Autodesk Inventor part; units mm, degrees
ref_plane "YZ Plane" through (0, 0, 0) normal (1, 0, 0) x (0, 1, 0)
ref_plane "XZ Plane" through (0, 0, 0) normal (0, 1, 0) x (-1, 0, 0)
ref_plane "XY Plane" through (0, 0, 0) normal (0, 0, 1) x (1, 0, 0)
sketch "Sketch1" plane through (0, 0, 0) normal (0, 1, 0) x (-1, 0, 0)
  line L0 (40.7614, 52.7865) -> (-35.4386, 52.7865)
  line L1 (-35.4386, 52.7865) -> (-35.4386, -99.6135)
  line L2 (-35.4386, -99.6135) -> (40.7614, -99.6135)
  line L3 (40.7614, -99.6135) -> (40.7614, 52.7865)
  circle A0 centre (2.6614, -23.4135) radius 25.4
  point P0 (0, 0)
  dimension "d0" = 152.4
  dimension "d1" = 76.2
  dimension "d2" = 50.8
  dimension "d5" = 76.2
  dimension "d6" = 38.1
extrude "Extrusion1" add sketch "Sketch1" along normal blind 12.7
sketch "Sketch2" plane through (-40.7614, 0, 52.7865) normal (0, 0, 1) x (1, 0, 0)
  line L0 (18.073, 9.7491) -> (58.127, 9.7491)
  line L1 (58.127, 9.7491) -> (58.127, 2.9509)
  line L2 (58.127, 2.9509) -> (18.073, 2.9509)
  line L3 (18.073, 2.9509) -> (18.073, 9.7491)
  line L4 (0, 12.7) -> (76.2, 12.7)
  line L5 (76.2, 0) -> (76.2, 12.7)
  line L6 (0, 0) -> (76.2, 0)
  line L7 (0, 0) -> (0, 12.7)
  point P0 (40.7614, 0)
  dimension "d9" = 2.9509
  dimension "d10" = 18.073
  dimension "d12" = 2.9509
  dimension "d13" = 18.073
extrude "Extrusion2" cut sketch "Sketch2" against normal up to surface (152.4 mm away) contours L0 L1 L2 L3
equation "\"d1\" = 0.5 * d0"
equation "\"d5\" = 0.5 * d0"
equation "\"d6\" = 0.5 * d1"
equation "\"d12\" = d9"
equation "\"d13\" = d10"
properties part number "Peg toy top"
Source: CAD feature listing. Evaluate the final solid. Frame: model axes, mm. A direction names the side the tool comes from. Coordinates: 2 decimals unless noted, no trailing zeros. Loops run counter-clockwise (first coordinate to the right, second up) from the corner with the lowest first, then second, coordinate; pieces in that order, holes last. Notation, with made-up numbers: M -12.75,69 L 33.25,69 A20 ccw 33.25,100 Z; hole C -19,17.5 d11. An arc over 180 degrees is marked long. Use a Markdown table: item, result. Add a question column.
Q1. Section query A-A, the plane y = 6.75. Return loops of the section in (x, z), and give its area (3 significant figures).
Q2. First-contact query: pin 1 (1 mm diameter, centred on x = -11.5, y = 4, fed in from -Z). Flat tip, straight axial feed; report the tip coordinate or a pass-through.
Q3. Material intervals for L1, parallel to X at y = 1, z = -24; L2, parallel to X at y = 4.5, z = -93; L3, parallel to Y at x = 13, z = -80.5, sorted ascending.
Q4. Section query C-C, the plane x = 3. Return loops of the section in (y, z).
Q5. Section query D-D, the plane x = -16. Return loops of the section in (y, z), and give its area (3 significant figures).
Q6. Section query B-B, the plane z = 33.5. Return loops of the section in (x, y).
Q7. Draft query along Y for faces 3 (the flat face through (23, 12.7, -22)), 4 (the flat face through (35.439, 6, -22)), 5 (the flat face through (-22.688, 6, 23)), 6 (the flat face through (17.366, 6, 23)). Return one class per face: pulls with the +Y half, pulls with the -Y half, needs draft (parallel to the pull), parting line crosses it, or undercut.
Q8. Access query for faces 1 (the cylindrical face through (-14.38, 10.49, -0.88)), 2 (the flat face through (-22.688, 6, -69)). Directions: +Z, -Z, +X, -X, +Y, -Y. A direction counts if a zero-diameter tool reaches every point of the face in a straight line with its end or side. Return the directions, or none.
Result:
| question | item | result |
|---|---|---|
| 1 | outline | M -40.76,-99.61 L -22.69,-99.61 L -22.69,-39.04 A25.4 cw -22.69,-7.79 L -22.69,52.79 L -40.76,52.79 Z; M 17.37,-99.61 L 35.44,-99.61 L 35.44,52.79 L 17.37,52.79 L 17.37,-7.79 A25.4 cw 17.37,-39.04 Z |
| 1 | area | 5,280 mm2 |
| 2 | pin 1 | passes through |
| 3 | L1 | x = -40.76 to -28.05, 22.73 to 35.44 |
| 3 | L2 | x = -40.76 to -22.69, 17.37 to 35.44 |
| 3 | L3 | y = 0 to 2.95, 9.75 to 12.7 |
| 4 | outline | M 0,-99.61 L 2.95,-99.61 L 2.95,-48.17 L 0,-48.17 Z; M 0,1.35 L 2.95,1.35 L 2.95,52.79 L 0,52.79 Z; M 9.75,-99.61 L 12.7,-99.61 L 12.7,-48.17 L 9.75,-48.17 Z; M 9.75,1.35 L 12.7,1.35 L 12.7,52.79 L 9.75,52.79 Z |
| 5 | outline | M 0,-99.61 L 2.95,-99.61 L 2.95,-45.03 L 0,-45.03 Z; M 0,-1.8 L 2.95,-1.8 L 2.95,52.79 L 0,52.79 Z; M 9.75,-99.61 L 12.7,-99.61 L 12.7,-45.03 L 9.75,-45.03 Z; M 9.75,-1.8 L 12.7,-1.8 L 12.7,52.79 L 9.75,52.79 Z |
| 5 | area | 644 mm2 |
| 6 | outline | M -40.76,0 L 35.44,0 L 35.44,12.7 L -40.76,12.7 Z; hole M -22.69,2.95 L 17.37,2.95 L 17.37,9.75 L -22.69,9.75 Z |
| 7 | face 3 | pulls with the +Y half |
| 7 | face 4 | needs draft |
| 7 | face 5 | undercut |
| 7 | face 6 | undercut |
| 8 | face 1 | +Y, -Y |
| 8 | face 2 | +Z, -Z |
